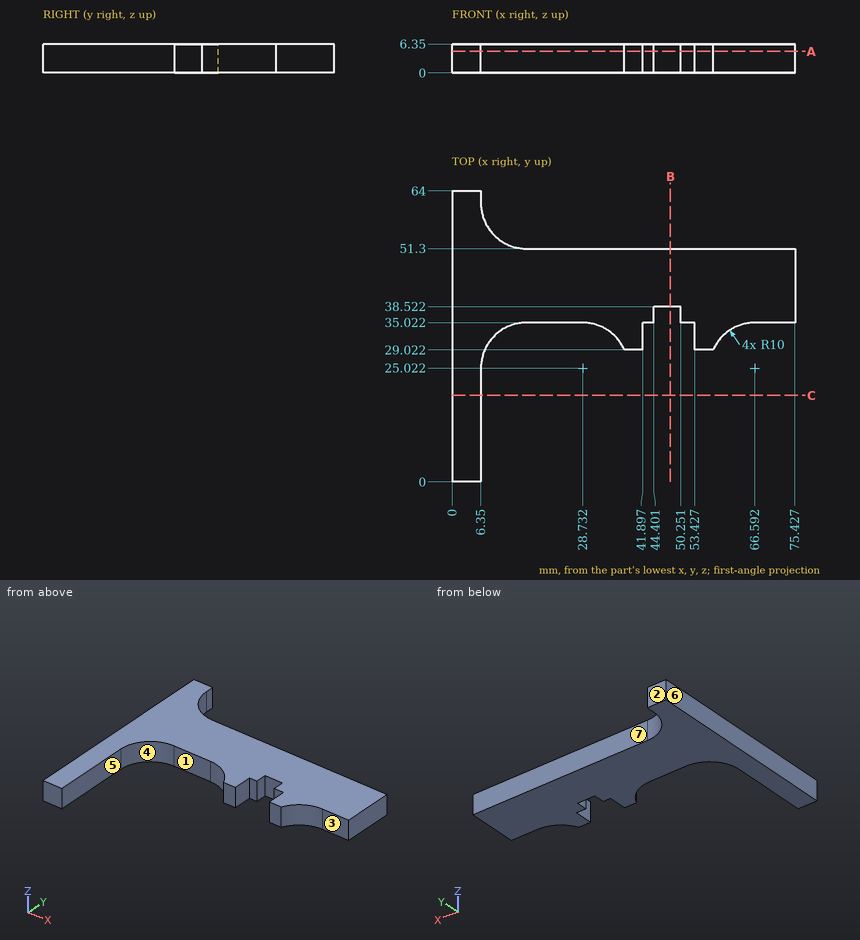
Source: three-view drawing plus pictorial views. Frame: mm from the lowest corner of the part. A direction names the side the tool comes from. Round coordinates to 2 decimals unless told otherwise and drop trailing zeros. Loops run counter-clockwise (first coordinate to the right, second up) from the corner with the lowest first, then second, coordinate; pieces in that order, holes last. Notation, with made-up numbers: M 2,88 L 29,88 A26 ccw 29,117 Z; hole C -24,-6.75 d5. An arc over 180 degrees is marked long. Put each result on its own line as item: value.
(1) Section B-B, the plane x = 48. Return loops of the section in (y, z).
Solutions:
outline: M 38.52,0 L 51.3,0 L 51.3,6.35 L 38.52,6.35 Z
(2) Section C-C, the plane y = 19. Return loops of the section in (x, z), and give its area (3 significant figures).
Solutions:
outline: M 0,0 L 6.35,0 L 6.35,6.35 L 0,6.35 Z
area: 40.3 mm²
(3) Pull-direction query (X, two-part tool) for the marked faces 4, 5, 6 and 7; classes: released by +X, released by -X, zero draft, split by the parting line, or undercut.
Solutions:
face 4: undercut
face 5: released by +X
face 6: released by -X
face 7: zero draft
(4) Access query for the marked faces 1, 2 and 3. Directions: +Z, -Z, +X, -X, +Y, -Y. A direction counts if a zero-diameter tool reaches every point of the face in a straight line with its end or side. Return the directions, or none.
Solutions:
face 1: +Z, -Z, -Y
face 2: +Z, -Z, +X, -X, +Y
face 3: +Z, -Z, +X, -Y
(5) Section A-A, the plane z = 4.75. Return loops of the section in (x, y), and give its area (3 significant figures).
Solutions:
outline: M 0,0 L 6.35,0 L 6.35,25.02 A10 cw 16.35,35.02 L 28.73,35.02 A10 cw 37.9,29.02 L 41.9,29.02 L 41.9,35.02 L 44.4,35.02 L 44.4,38.52 L 50.25,38.52 L 50.25,35.02 L 53.43,35.02 L 53.43,29.02 L 57.43,29.02 A10 cw 66.59,35.02 L 75.43,35.02 L 75.43,51.3 L 16.35,51.3 A10 cw 6.35,61.3 L 6.35,64 L 0,64 Z
area: 1,630 mm²
(6) Ray query, line 1 (Y direction, x = 54, z = 4.5); line 2 (Y direction, x = 27.5, z = 6); line 3 (X direction, y = 11, z = 1.25). Return the intervals inside material, ascending. Write a range as [from, to].
Solutions:
line 1: [29.02, 51.3]
line 2: [35.02, 51.3]
line 3: [0, 6.35]
(7) First-contact query: pin 1 (0.8 mm diameter, centred on x = 44, z = 4, fed in from -Y); pin 2 (3 mm diameter, centred on x = 39.5, z = 2.5, fed in from -Y); pin 3 (1.8 mm diameter, centred on x = 46, z = 2.5, fed in from -Y). Flat tips, straight axial feed; report the tip coordinate or a pass-through.
Solutions:
pin 1: y = 35.02
pin 2: y = 29.02
pin 3: y = 38.52
